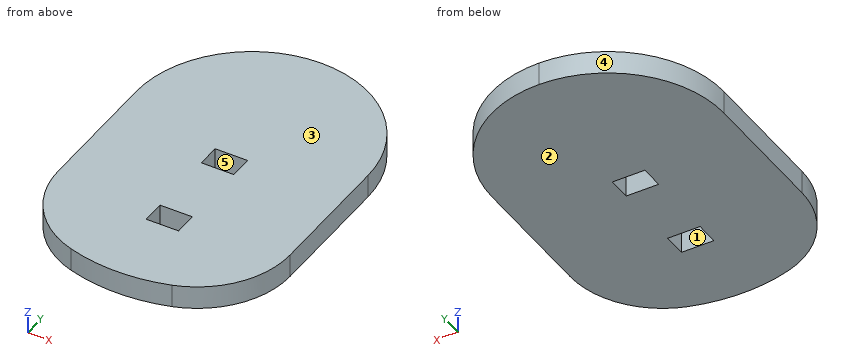
```python
from build123d import *

# Parameters (mm, degrees)
SKETCH1_R           = 37
BOSS_EXTRUDE1_DEPTH = 5
CUT_EXTRUDE3_START  = -10
CUT_EXTRUDE3_DEPTH  = 10
FILLET1_R           = 25
FILLET2_R           = 20
SKETCH11_W          = 7
SKETCH11_H          = 5
CUT_EXTRUDE4_DEPTH  = 10


with BuildPart() as part:
    # Sketch1 → Boss-Extrude1 (new body)
    with BuildSketch(Plane.XY):
        Circle(SKETCH1_R)
    extrude(amount=BOSS_EXTRUDE1_DEPTH)

    # Sketch10 → Cut-Extrude3 (cut)
    with BuildSketch(Plane.XY.offset(5).offset(CUT_EXTRUDE3_START)):
        with BuildLine():
            Line((-25, 27.276363394), (-25, -27.276363394))
            ThreePointArc((-25, -27.276363394), (-37, 0), (-25, 27.276363394))
        make_face()
        with BuildLine():
            Line((25, -27.276363394), (25, 27.276363394))
            ThreePointArc((25, 27.276363394), (37, 0), (25, -27.276363394))
        make_face()
    extrude(amount=CUT_EXTRUDE3_DEPTH, mode=Mode.SUBTRACT)

    # Fillet1
    fillet1_edges = [part.edges().sort_by_distance(p)[0] for p in [
        (-25, 27.276363394, 2.5),
        (25, 27.276363394, 2.5),
    ]]
    fillet(fillet1_edges, radius=FILLET1_R - 0.0001)  # a hair under: the kernel refuses the full size

    # Fillet2
    fillet2_edges = [part.edges().sort_by_distance(p)[0] for p in [
        (-25, -27.276363394, 2.5),
        (25, -27.276363394, 2.5),
    ]]
    fillet(fillet2_edges, radius=FILLET2_R)

    # Sketch11 → Cut-Extrude4 (cut)
    with BuildSketch(Plane.XY.offset(5)):
        with Locations((0, 2)):
            Rectangle(SKETCH11_W, SKETCH11_H)
        with Locations((0, -18)):
            Rectangle(SKETCH11_W, SKETCH11_H)
    extrude(amount=-CUT_EXTRUDE4_DEPTH, mode=Mode.SUBTRACT)


solid = part.part
```
Geometry check sheet. Reference: the model listing, model coordinates, mm. Face numbers are marked on the shaded views. A direction names the side the tool comes from. Round coordinates to 2 decimals unless told otherwise and drop trailing zeros. Loops run counter-clockwise (first coordinate to the right, second up) from the corner with the lowest first, then second, coordinate; pieces in that order, holes last. Notation, with made-up numbers: (51.25, 4) - (87.25, 4) arc R33 ccw to (87.25, 42) - close; hole circle Ø4 at (2.5, 65). An arc over 180 degrees is marked (long way). Use a Markdown table: item, result.
Q1. Material ranges on line 1 (Y direction, x = 0.5, z = 0.4) (3 decimals); line 2 (X direction, y = 1, z = 3.55); line 3 (Y direction, x = -13, z = 3.2), recorded low to high.
Solutions:
| item | result |
|---|---|
| line 1 | y = -36.997 to -20.5, -15.5 to -0.5, 4.5 to 36.995 |
| line 2 | x = -25 to -3.5, 3.5 to 25 |
| line 3 | y = -34.58 to 33.35 |
Q2. Go/stop test with flat-tipped pins: P1, Ø1.5, axis at y = -19, z = 2.5, coming from the -X side; P2, Ø1, axis at x = -3.5, z = 1.5, coming from the -Y side; P3, Ø3, axis at x = 7, z = 3.5, coming from the +Y side. Record where each tip stops, or that it passes through.
Solutions:
| item | result |
|---|---|
| P1 | stops at x = -24.9 |
| P2 | stops at y = -36.88 |
| P3 | stops at y = 36.39 |
Q3. Cross-section at B-B on y = -18. Record the cut outline in (x, z), plus the area to 3 significant figures.
Solutions:
| item | result |
|---|---|
| outline | (-24.92, 0) - (-3.5, 0) - (-3.5, 5) - (-24.92, 5) - close; (3.5, 0) - (24.92, 0) - (24.92, 5) - (3.5, 5) - close |
| area | 214 mm2 |
Q4. Access from +Z, -Z, +X, -X, +Y, -Y to the whole of each face (thin tool, end or side, straight path). Record for the marked faces 1 and 2.
Solutions:
| item | result |
|---|---|
| face 1 | +Z, -Z |
| face 2 | -Z, +X, -X, +Y, -Y |
Q5. Cross-section at C-C on x = 12. Record the cut outline in (y, z), plus the area to 3 significant figures.
Solutions:
| item | result |
|---|---|
| outline | (-34.98, 0) - (33.93, 0) - (33.93, 5) - (-34.98, 5) - close |
| area | 345 mm2 |
Q6. Draft check along X on the marked faces 3, 4 and 5. Enter one of: released by +X, released by -X, zero draft, split by the parting line, or undercut.
Solutions:
| item | result |
|---|---|
| face 3 | zero draft |
| face 4 | released by -X |
| face 5 | undercut |
Q7. Cross-section at D-D on y = -26. Record the cut outline in (x, z), plus the area to 3 significant figures.
Solutions:
| item | result |
|---|---|
| outline | (-22.46, 0) - (22.46, 0) - (22.46, 5) - (-22.46, 5) - close |
| area | 225 mm2 |
Q8. Cross-section at A-A on z = 0.8. State how many separate pieces and enclosed holes the cut face has, plus the area to 3 significant figures.
Solutions:
| item | result |
|---|---|
| separate pieces | 1 |
| enclosed holes | 2 |
| area | 3,160 mm2 |
